Here's how the part is built. I have some questions about the finished solid (model axes, mm). A direction names the side the tool comes from. Coordinates: 2 decimals unless noted, no trailing zeros. Write each loop counter-clockwise with the first axis right and the second up, starting at its lowest first coordinate (ties: lowest second). Pieces come first, ordered by that corner, then holes. Notation, with made-up numbers: (-26, 38.25) -> (12, 38.25) arc R20 ccw to (12, 44.25) -> close; hole circle Ø1 at (10, -29.75). An arc over 180 degrees is marked (long way). Answer in a Markdown table with one row per item. Add a question column.
from build123d import *

# Parameters (mm, degrees)
BOSS_EXTRUDE1_DEPTH = 2
BOSS_EXTRUDE2_DEPTH = 4.4
BOSS_EXTRUDE9_DEPTH = 10
FILLET1_R           = 10
SKETCH6_W           = 13.75
SKETCH6_H           = 1
CUT_EXTRUDE2_DEPTH  = 10


with BuildPart() as part:
    # Sketch1 → Boss-Extrude1 (new body)
    with BuildSketch(Plane(origin=(0, 0, 0), x_dir=(1, 0, 0), z_dir=(0, 1, 0))):
        with BuildLine():
            Line((-43.608869745, 4.4), (-27.608869745, 4.4))
            ThreePointArc((-27.608869745, 4.4), (-26.964504664, 2.844365081), (-25.408869745, 2.2))
            Line((-25.408869745, 2.2), (-25.408869745, -4.4))
            Line((-25.408869745, -4.4), (-43.608869745, -4.4))
            Line((-43.608869745, -4.4), (-43.608869745, 4.4))
        make_face()
    extrude(amount=BOSS_EXTRUDE1_DEPTH)

    # Sketch2 → Boss-Extrude2 (add)
    with BuildSketch(Plane.XZ):
        Polygon((-39.358869745, -4.4), (-27.608869745, -4.4), (-27.608869745, -2.8), (-39.358869745, -2.8), (-39.358869745, 4.4), (-43.608869745, 4.4), (-43.608869745, -4.4), align=None)
    extrude(amount=BOSS_EXTRUDE2_DEPTH)

    # Sketch3 → Boss-Extrude9 (add)
    with BuildSketch(Plane.XZ.offset(4.4)):
        Polygon((-41.358869745, 2.8), (-25.408869745, 2.8), (-25.408869745, 0.5), (-39.358869745, 0.5), (-39.358869745, -2), (-27.608869745, -2), (-27.608869745, -2.8), (-27.608869745, -3.8), (-41.358869745, -3.8), (-41.358869745, -2.8), align=None)
    extrude(amount=BOSS_EXTRUDE9_DEPTH)

    # Fillet1
    # the kernel refuses this fillet: 10 mm, written as the material it adds along each edge
    with BuildSketch(Plane(origin=(-27.608869745, -4.4, -2.8), x_dir=(0, 1, 0), z_dir=(-1, 0, 0))) as fillet1_piece_1_section:
        with BuildLine():
            CenterArc((3.919183588, -10), FILLET1_R, 90, 23.073918066)
            Line((0, -0.8), (0, 0))
            Line((0, 0), (3.919183588, 0))
        make_face()
    fillet1_piece_1 = extrude(amount=21.547958971, mode=Mode.PRIVATE)
    fillet1_piece_1 = split(fillet1_piece_1, bisect_by=Plane(origin=(-41.358869745, -4.4, -2.8), z_dir=(1, 0, 0)), keep=Keep.TOP, mode=Mode.PRIVATE)
    add(fillet1_piece_1)

    # Sketch6 → Cut-Extrude2 (cut)
    with BuildSketch(Plane.XZ.offset(14.4)):
        with Locations((-34.483869745, -3.3)):
            Rectangle(SKETCH6_W, SKETCH6_H)
    extrude(amount=-CUT_EXTRUDE2_DEPTH, mode=Mode.SUBTRACT)


solid = part.part
Q1. Imagine slicing it at D-D on y = 1.25. Please give me the cut outline in (x, z), plus the area to 3 significant figures.
Q2. I need wall thicknesses on line 1 (Z direction, x = -29, y = -7.25); line 2 (Y direction, x = -37.75, z = 0.75); line 3 (X direction, y = -12.75, z = -2.5). Which ranges of each line are inside material? Lowest first, please. Write a range as [from, to].
Q3. For faces 1 (the flat face through (-34, -9, -2)), 2 (the flat face through (-41.359, -9, 0)), 3 (the flat face through (-32, -4.4, 2)), 4 (the flat face through (-35, -9, -2.8)), 5 (the flat face through (-33, -9, 2.8)), which set-ups out of +Z, -Z, +X, -X, +Y, -Y let a thin tool reach every point of the face, with its end or its side?
Q4. I'm going to push flat-ended pins straight in: P1, Ø3, axis at x = -37, y = -11.5, coming from the +Z side; P2, Ø5, axis at x = -35.5, y = -7.5, coming from the -Z side; P3, Ø3, axis at y = -9.5, z = -0.5, coming from the -X side. Where does each tip first touch, or does it pass through?
Q5. Imagine slicing it at B-B on z = 2.25. Please give me the cut outline in (x, y).
Q6. Imagine slicing it at C-C on y = -5.25. Please give me the cut outline in (x, z), plus the area to 3 significant figures.
Q7. Imagine slicing it at A-A on x = -30.5. Please give me the cut outline in (y, z), plus the area to 3 significant figures.
Result sheet:
| question | item | result |
|---|---|---|
| 1 | outline | (-43.61, -4.4) -> (-27.61, -4.4) arc R2.2 cw to (-25.41, -2.2) -> (-25.41, 4.4) -> (-43.61, 4.4) -> close |
| 1 | area | 156 mm^2 |
| 2 | line 1 | z = [-2.8, -2], [0.5, 2.8] |
| 2 | line 2 | y = [-14.4, -4.4], [0, 2] |
| 2 | line 3 | x = [-41.36, -27.61] |
| 3 | face 1 | +X, -Y |
| 3 | face 2 | +Z, -Z, -X, -Y |
| 3 | face 3 | +Z, +X |
| 3 | face 4 | -Z, +X, -X, -Y |
| 3 | face 5 | +Z, +X, -X, -Y |
| 4 | P1 | stops at z = 2.8 |
| 4 | P2 | stops at z = -2.8 |
| 4 | P3 | stops at x = -41.36 |
| 5 | outline | (-43.61, -4.4) -> (-41.36, -4.4) -> (-41.36, -14.4) -> (-25.41, -14.4) -> (-25.41, -4.4) -> (-39.36, -4.4) -> (-39.36, 0) -> (-25.41, 0) -> (-25.41, 2) -> (-43.61, 2) -> close |
| 6 | outline | (-41.36, -2.8) -> (-27.61, -2.8) -> (-27.61, -2) -> (-39.36, -2) -> (-39.36, 0.5) -> (-25.41, 0.5) -> (-25.41, 2.8) -> (-41.36, 2.8) -> close |
| 6 | area | 52.7 mm^2 |
| 7 | outline | (-14.4, -2.8) -> (-4.4, -2.8) -> (-4.4, -4.4) -> (2, -4.4) -> (2, 4.4) -> (0, 4.4) -> (0, -2.8) -> (-0.48, -2.8) arc R10 cw to (-4.4, -2) -> (-14.4, -2) -> close; (-14.4, 0.5) -> (-4.4, 0.5) -> (-4.4, 2.8) -> (-14.4, 2.8) -> close |
| 7 | area | 56.7 mm^2 |
